Read the model definition and answer for the solid it produces. Units are mm, in the model's axes. A direction names the side the tool comes from. Coordinates: 2 decimals unless noted, no trailing zeros. Loops run counter-clockwise (first coordinate to the right, second up) from the corner with the lowest first, then second, coordinate; pieces in that order, holes last. Notation, with made-up numbers: (33, 67.5) - (81, 67.5) arc R8 ccw to (81, 75.5) - close; hole circle Ø7 at (-3.5, 49.25). An arc over 180 degrees is marked (long way). Use CSV: the item, a comma, the result in double quotes.
```python
from build123d import *

# Parameters (mm, degrees)
SKETCH_1_W                  = 15
SKETCH_1_H                  = 15
EXTRUDE_1_DEPTH             = 30
CHAMFER_1_SIZE              = 5
HOLE_WIZARD_M3_2_AT_2_COUNT = 2
HOLE_WIZARD_M3_2_AT_2_PITCH = 9.899494937
SKETCH_5_W                  = 2
SKETCH_5_H                  = 30
CUT_EXTRUDE_1_DEPTH         = 2
SKETCH_6_W                  = 30
SKETCH_6_H                  = 2
CUT_EXTRUDE_2_DEPTH         = 2


with BuildPart() as part:
    # 草图1 → 凸台-拉伸1 (new body)
    with BuildSketch(Plane.XY):
        Rectangle(SKETCH_1_W, SKETCH_1_H)
    extrude(amount=EXTRUDE_1_DEPTH)

    # 倒角1
    chamfer_1_edges = [part.edges().sort_by_distance(p)[0] for p in [
        (-7.5, 7.5, 15),
    ]]
    chamfer(chamfer_1_edges, length=CHAMFER_1_SIZE)

    # 草图3 → M3 螺纹孔2 (revolve, cut)
    with BuildSketch(Plane(origin=(-3.5, -3.5, 30), x_dir=(0, -1, 0), z_dir=(1, 0, 0))):
        Polygon((0, 0), (0, 8.251075774), (1.25, 7.5), (1.25, 0), align=None)
    hole_wizard_m3_2 = revolve(axis=Axis((-3.5, -3.5, 36.35), (0, 0, -1)), mode=Mode.SUBTRACT)

    # M3 螺纹孔2 at 2: M3 螺纹孔2 ×2
    with Locations(*[Vector(0.707106781, 0.707106781, 0) * (i * HOLE_WIZARD_M3_2_AT_2_PITCH) for i in range(1, HOLE_WIZARD_M3_2_AT_2_COUNT)]):
        add(hole_wizard_m3_2, mode=Mode.SUBTRACT)

    # 镜向1: M3 螺纹孔2 across plane
    add(hole_wizard_m3_2.mirror(Plane(origin=(0, 0, 15), x_dir=(1, 0, 0), z_dir=(0, 0, -1))), mode=Mode.SUBTRACT)

    # 镜向1 copy 1 sketch → 镜向1 copy 1 (revolve, cut)
    with BuildSketch(Plane(origin=(3.5, 3.5, 0), x_dir=(0, -1, 0), z_dir=(1, 0, 0))):
        Polygon((0, 0), (0, -8.251075774), (1.25, -7.5), (1.25, 0), align=None)
    revolve(axis=Axis((3.5, 3.5, -6.35), (0, 0, -1)), mode=Mode.SUBTRACT)

    # 草图5 → 切除-拉伸1 (cut)
    with BuildSketch(Plane(origin=(0, 7.5, 0), x_dir=(1, 0, 0), z_dir=(0, 1, 0))):
        with Locations((6.5, -15)):
            Rectangle(SKETCH_5_W, SKETCH_5_H)
    extrude(amount=-CUT_EXTRUDE_1_DEPTH, mode=Mode.SUBTRACT)

    # 草图6 → 切除-拉伸2 (cut)
    with BuildSketch(Plane.ZY.offset(7.5)):
        with Locations((15, -6.5)):
            Rectangle(SKETCH_6_W, SKETCH_6_H)
    extrude(amount=-CUT_EXTRUDE_2_DEPTH, mode=Mode.SUBTRACT)


solid = part.part
```
Q1. A tool of negligible diameter and unlimited length cuts with its end or side. For faces 5 (the face through (3.45, 4.75, 26.3)), 6 (the face through (5.5, 7, 15)), 7 (the face through (4.609, 2.923, 3.698)), from which of +Z, -Z, +X, -X, +Y, -Y can it reach the whole face along a straight path? Write none if from no direction.
Reported:
face 5,"+Z"
face 6,"+Z, -Z, +X, +Y"
face 7,"-Z"
Q2. The part is cut by section C-C on y = -6. Determine the outline of the cut face in (x, z), and give its area (3 significant figures).
Reported:
outline,"(-5.5, 0) - (7.5, 0) - (7.5, 30) - (-5.5, 30) - close"
area,"390 mm²"
Q3. Given P1, Ø4, axis at x = -3.5, y = -3.5, coming from the +Z side; P2, Ø0.6, axis at y = -6, z = 22, coming from the -X side; P3, Ø2, axis at x = 3.5, y = 3.5, coming from the -Z side; P4, Ø0.6, axis at x = 6.5, z = 18.5, coming from the +Y side, each flat-ended and moving along its own axis, determine where each tip first touches the part or whether it passes through.
Reported:
P1,"stops at z = 30"
P2,"stops at x = -5.5"
P3,"stops at z = 7.65"
P4,"stops at y = 5.5"
Q4. For a pull along Y with two mould halves and no side action, classify faces 1 (the face through (-7, -5.5, 15)), 2 (the face through (3.285, 3.528, 21.879)), 3 (the face through (3.35, 3.66, 8.12)), 4 (the face through (7.5, -1, 15)) as +Y half, -Y half, draft (parallel to the pull), parting line (faces both ways), or undercut.
Reported:
face 1,"-Y half"
face 2,"undercut"
face 3,"undercut"
face 4,"draft"
Q5. The part is cut by section A-A on z = 5.5. Determine the outline of the cut face in (x, y).
Reported:
outline,"(-7.5, -5.5) - (-5.5, -5.5) - (-5.5, -7.5) - (7.5, -7.5) - (7.5, 5.5) - (5.5, 5.5) - (5.5, 7.5) - (-2.5, 7.5) - (-7.5, 2.5) - close; hole circle Ø2.5 at (-3.5, -3.5); hole circle Ø2.5 at (3.5, 3.5)"
Q6. Find the intervals of material crossed by probe 1 along Y at (x, z) = (3.5, 24.5); probe 2 along X at (y, z) = (-3.5, 26); probe 3 along X at (y, z) = (-6, 14.75), in increasing order. Write a range as [from, to].
Reported:
probe 1,"y = [-7.5, 2.25], [4.75, 7.5]"
probe 2,"x = [-7.5, -4.75], [-2.25, 7.5]"
probe 3,"x = [-5.5, 7.5]"
Q7. The part is cut by section B-B on x = 6.75. Determine the outline of the cut face in (y, z).
Reported:
outline,"(-7.5, 0) - (5.5, 0) - (5.5, 30) - (-7.5, 30) - close"
